from build123d import *

# Parameters (mm, degrees)
SKETCH1_W             = 106.985396655
SKETCH1_H             = 86
SKETCH1_R             = 3.5
SKETCH1_R_2           = 1.5
BOSS_EXTRUDE1_DEPTH   = 3
SKETCH3_R             = 3.5
BOSS_EXTRUDE2_DEPTH   = 7
BOSS_EXTRUDE2_2_DEPTH = 7
BOSS_EXTRUDE2_3_DEPTH = 7
BOSS_EXTRUDE2_4_DEPTH = 7
SKETCH4_R             = 3.5
BOSS_EXTRUDE3_DEPTH   = 3
SKETCH5_R             = 1.25
CUT_EXTRUDE1_DEPTH    = 7
SKETCH6_R             = 2.5
CUT_EXTRUDE2_DEPTH    = 2


with BuildPart() as part:
    # Sketch1 → Boss-Extrude1 (new body)
    with BuildSketch(Plane(origin=(0, 0, 0), x_dir=(1, 0, 0), z_dir=(0, 1, 0))):
        with Locations((-33.080324924, 0)):
            Rectangle(SKETCH1_W, SKETCH1_H)
        with Locations((11, 36)):
            Circle(SKETCH1_R, mode=Mode.SUBTRACT)
        with Locations((-7, 38)):
            Circle(SKETCH1_R_2, mode=Mode.SUBTRACT)
        with Locations((-26.5, 38)):
            Circle(SKETCH1_R_2, mode=Mode.SUBTRACT)
        with Locations((-75, -22)):
            Circle(SKETCH1_R, mode=Mode.SUBTRACT)
        with Locations((-33.5, -38)):
            Circle(SKETCH1_R_2, mode=Mode.SUBTRACT)
        with Locations((-33.5, -28)):
            Circle(SKETCH1_R_2, mode=Mode.SUBTRACT)
        with Locations((-26.5, -38)):
            Circle(SKETCH1_R_2, mode=Mode.SUBTRACT)
        with Locations((-26.5, -28)):
            Circle(SKETCH1_R_2, mode=Mode.SUBTRACT)
        with Locations((-7, -38)):
            Circle(SKETCH1_R_2, mode=Mode.SUBTRACT)
        with Locations((0, -38)):
            Circle(SKETCH1_R_2, mode=Mode.SUBTRACT)
        with Locations((-7, -28)):
            Circle(SKETCH1_R_2, mode=Mode.SUBTRACT)
        with Locations((0, -28)):
            Circle(SKETCH1_R_2, mode=Mode.SUBTRACT)
        with Locations((11, -22)):
            Circle(SKETCH1_R, mode=Mode.SUBTRACT)
        Polygon((1.724967874, 23), (1.724967874, -22), (1.724967874, -23), (-69.131444758, -23), (-69.131444758, 23), align=None, mode=Mode.SUBTRACT)
        with Locations((-75, 36)):
            Circle(SKETCH1_R, mode=Mode.SUBTRACT)
        with Locations((-33.5, 28)):
            Circle(SKETCH1_R_2, mode=Mode.SUBTRACT)
        with Locations((-33.5, 38)):
            Circle(SKETCH1_R_2, mode=Mode.SUBTRACT)
        with Locations((-26.5, 28)):
            Circle(SKETCH1_R_2, mode=Mode.SUBTRACT)
        with Locations((-7, 28)):
            Circle(SKETCH1_R_2, mode=Mode.SUBTRACT)
        with Locations((0, 28)):
            Circle(SKETCH1_R_2, mode=Mode.SUBTRACT)
        with Locations((0, 38)):
            Circle(SKETCH1_R_2, mode=Mode.SUBTRACT)
    extrude(amount=BOSS_EXTRUDE1_DEPTH)



with BuildPart() as body_2:
    # Sketch3 → Boss-Extrude2 (new body)
    with BuildSketch(Plane(origin=(0, 3, 0), x_dir=(1, 0, 0), z_dir=(0, 1, 0))):
        with Locations((-75, -22)):
            Circle(SKETCH3_R)
    extrude(amount=BOSS_EXTRUDE2_DEPTH)


with BuildPart() as body_3:
    # Sketch3 → Boss-Extrude2 2 (new body)
    with BuildSketch(Plane(origin=(0, 3, 0), x_dir=(1, 0, 0), z_dir=(0, 1, 0))):
        with Locations((11, -22)):
            Circle(SKETCH3_R)
    extrude(amount=BOSS_EXTRUDE2_2_DEPTH)


with BuildPart() as body_4:
    # Sketch3 → Boss-Extrude2 3 (new body)
    with BuildSketch(Plane(origin=(0, 3, 0), x_dir=(1, 0, 0), z_dir=(0, 1, 0))):
        with Locations((11, 36)):
            Circle(SKETCH3_R)
    extrude(amount=BOSS_EXTRUDE2_3_DEPTH)


with BuildPart() as body_5:
    # Sketch3 → Boss-Extrude2 4 (new body)
    with BuildSketch(Plane(origin=(0, 3, 0), x_dir=(1, 0, 0), z_dir=(0, 1, 0))):
        with Locations((-75, 36)):
            Circle(SKETCH3_R)
    extrude(amount=BOSS_EXTRUDE2_4_DEPTH)


with BuildPart() as part_1:
    add(part.part)

    add(body_2.part)  # Boss-Extrude3 merges body 2

    add(body_3.part)  # Boss-Extrude3 merges body 3

    add(body_4.part)  # Boss-Extrude3 merges body 4

    add(body_5.part)  # Boss-Extrude3 merges body 5
    # Sketch4 → Boss-Extrude3 (add)
    with BuildSketch(Plane.XZ.offset(-3)):
        with Locations((-75, -36)):
            Circle(SKETCH4_R)
        with Locations((11, -36)):
            Circle(SKETCH4_R)
        with Locations((11, 22)):
            Circle(SKETCH4_R)
        with Locations((-75, 22)):
            Circle(SKETCH4_R)
    extrude(amount=BOSS_EXTRUDE3_DEPTH)

    # Sketch5 → Cut-Extrude1 (cut)
    with BuildSketch(Plane(origin=(0, 10, 0), x_dir=(1, 0, 0), z_dir=(0, 1, 0))):
        with Locations((11, 36)):
            Circle(SKETCH5_R)
        with Locations((11, -22)):
            Circle(SKETCH5_R)
        with Locations((-75, -22)):
            Circle(SKETCH5_R)
        with Locations((-75, 36)):
            Circle(SKETCH5_R)
    extrude(amount=-CUT_EXTRUDE1_DEPTH, mode=Mode.SUBTRACT)

    # Sketch6 → Cut-Extrude2 (cut)
    with BuildSketch(Plane(origin=(0, 10, 0), x_dir=(1, 0, 0), z_dir=(0, 1, 0))):
        with Locations((-75, 36)):
            Circle(SKETCH6_R)
        with Locations((11, 36)):
            Circle(SKETCH6_R)
        with Locations((-75, -22)):
            Circle(SKETCH6_R)
        with Locations((11, -22)):
            Circle(SKETCH6_R)
    extrude(amount=-CUT_EXTRUDE2_DEPTH, mode=Mode.SUBTRACT)


solid = part_1.part
Read the model definition and answer for the solid it produces. Units are mm, in the model's axes. A direction names the side the tool comes from. Round coordinates to 2 decimals unless told otherwise and drop trailing zeros. Loops run counter-clockwise (first coordinate to the right, second up) from the corner with the lowest first, then second, coordinate; pieces in that order, holes last.
Q1. Determine the mould class of faces 4 (the face through (13, 10, 24)), 5 (the face through (-7.325, 1.479, 39.464)), 6 (the face through (-86.573, 1, 1)), 7 (the face through (-75, 3, -36)) for opening direction X: released by +X, released by -X, zero draft, split by the parting line, or undercut.
Q2. Section A-A on y = 5.75 is taken. Write down the section's boundary in (x, z).
Q3. Section B-B on x = -29.5 is taken. Write down the section's boundary in (y, z), and give its area (3 significant figures).
Q4. Consider probe 1 along Z at (x, y) = (-75, 8.8); probe 2 along X at (y, z) = (1.3, 28); probe 3 along Z at (x, y) = (0, 1.7). Determine where each line is inside the solid, lowest interval first.
Q5. Section C-C on z = -28 is taken. Write down the section's boundary in (x, y).
Q6. Which of the six approach directions +Z, -Z, +X, -X, +Y, -Y give full straight-line access (tool end or side, diameter ignored) to faces 1 (the face through (-69.131, 1, 0)), 2 (the face through (-34, 1, -43)), 3 (the face through (10.01, 5.54, -35.24))?
Q7. Each of these flat-tipped pins is pushed along its axis until it touches: pin 1 (6 mm diameter, centred on x = -26, z = -29.5, fed in from -Y); pin 2 (3 mm diameter, centred on x = 11, z = -36, fed in from +Y); pin 3 (3.5 mm diameter, centred on x = 0, z = -38, fed in from +Y). Where does it stop, or does it pass through?
Q8. Section D-D on x = 0 is taken. Write down the section's boundary in (y, z), and give its area (3 significant figures).
Output:
1. face 4: zero draft
1. face 5: undercut
1. face 6: released by -X
1. face 7: undercut
2. outline: circle Ø7 at (-75, -36); circle Ø7 at (-75, 22); circle Ø7 at (11, -36); circle Ø7 at (11, 22); hole circle Ø2.5 at (-75, -36); hole circle Ø2.5 at (-75, 22); hole circle Ø2.5 at (11, -36); hole circle Ø2.5 at (11, 22)
3. outline: (0, -43) - (3, -43) - (3, -23) - (0, -23) - close; (0, 23) - (3, 23) - (3, 43) - (0, 43) - close
3. area: 120 mm2
4. probe 1: z = -39.5 to -38.5, -33.5 to -32.5, 18.5 to 19.5, 24.5 to 25.5
4. probe 2: x = -86.57 to -35, -32 to -28, -25 to -8.5, -5.5 to -1.5, 1.5 to 20.41
4. probe 3: z = -43 to -39.5, -36.5 to -29.5, -26.5 to -23, 23 to 26.5, 29.5 to 36.5, 39.5 to 43
5. outline: (-86.57, 0) - (-35, 0) - (-35, 3) - (-86.57, 3) - close; (-32, 0) - (-28, 0) - (-28, 3) - (-32, 3) - close; (-25, 0) - (-8.5, 0) - (-8.5, 3) - (-25, 3) - close; (-5.5, 0) - (-1.5, 0) - (-1.5, 3) - (-5.5, 3) - close; (1.5, 0) - (20.41, 0) - (20.41, 3) - (1.5, 3) - close
6. face 1: +Y, -Y
6. face 2: -Z, +X, -X, +Y, -Y
6. face 3: +Y
7. pin 1: stops at y = 0
7. pin 2: stops at y = 8
7. pin 3: stops at y = 3
8. outline: (0, -43) - (3, -43) - (3, -39.5) - (0, -39.5) - close; (0, -36.5) - (3, -36.5) - (3, -29.5) - (0, -29.5) - close; (0, -26.5) - (3, -26.5) - (3, -23) - (0, -23) - close; (0, 23) - (3, 23) - (3, 26.5) - (0, 26.5) - close; (0, 29.5) - (3, 29.5) - (3, 36.5) - (0, 36.5) - close; (0, 39.5) - (3, 39.5) - (3, 43) - (0, 43) - close
8. area: 84.0 mm2
